```python
from build123d import *

# Parameters (mm, degrees)
BASE_FLANGE1_START                           = -50
BASE_FLANGE1_DEPTH                           = 100
CSK_FOR_M5_COUNTERSUNK_FLAT_HEAD_SCR_2_COUNT = 2
CSK_FOR_M5_COUNTERSUNK_FLAT_HEAD_SCR_2_PITCH = 50
FILLET1_R                                    = 10


# Read off the part's stored shape, not the designer's step: Base-Flange1
with BuildPart() as part:
    # Base-Flange1 outline → Base-Flange1 (new body)
    with BuildSketch(Plane(origin=(0, 0, 0), x_dir=(0, 0, -1), z_dir=(1, 0, 0)).offset(BASE_FLANGE1_START)):
        with BuildLine():
            Line((-47.884076231, -4), (50, -4))
            Line((50, -4), (50, 0))
            Line((50, 0), (-47.884076231, 0))
            ThreePointArc((-47.884076231, 0), (-49.967854363, -0.182306964), (-51.988317951, -0.723688551))
            Line((-51.988317951, -0.723688551), (-100, -18.198511713))
            Line((-100, -18.198511713), (-98.631919427, -21.957282196))
            Line((-98.631919427, -21.957282196), (-50.620237378, -4.482459034))
            ThreePointArc((-50.620237378, -4.482459034), (-49.273261653, -4.121537976), (-47.884076231, -4))
        make_face()
    extrude(amount=BASE_FLANGE1_DEPTH)

    # Sketch8 → CSK for M5 Countersunk Flat Head Screw1 (revolve, cut)
    with BuildSketch(Plane(origin=(0, -4, 25), x_dir=(0, 0, -1), z_dir=(1, 0, 0))):
        Polygon((0, 0), (0, 4), (2.75, 4), (2.75, 3.25), (6, 0), align=None)
    csk_for_m5_countersunk_flat_head_screw1 = revolve(axis=Axis((0, -10.35, 25), (0, 1, 0)), mode=Mode.SUBTRACT)

    # CSK for M5 Countersunk Flat Head Scr 2: CSK for M5 Countersunk Flat Head Screw1 ×2
    with Locations(*[(0, 0, -i * CSK_FOR_M5_COUNTERSUNK_FLAT_HEAD_SCR_2_PITCH) for i in range(1, CSK_FOR_M5_COUNTERSUNK_FLAT_HEAD_SCR_2_COUNT)]):
        add(csk_for_m5_countersunk_flat_head_screw1, mode=Mode.SUBTRACT)

    # Fillet1
    fillet1_edges = [part.edges().sort_by_distance(p)[0] for p in [
        (50, -20.077896954, 99.315959714),
        (50, -2, -50),
        (-50, -20.077896954, 99.315959714),
        (-50, -2, -50),
    ]]
    fillet(fillet1_edges, radius=FILLET1_R)


solid = part.part
```
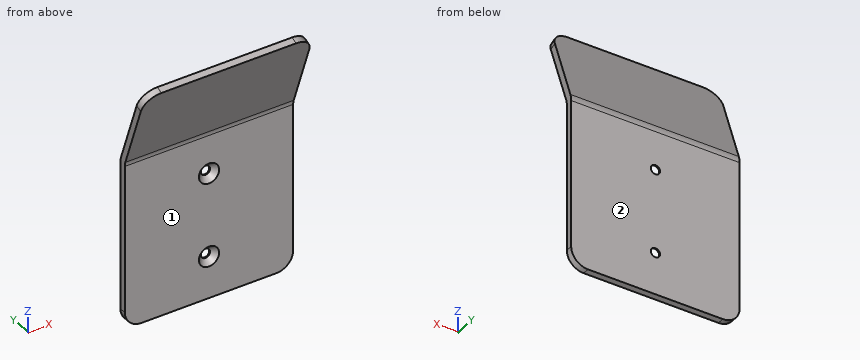
Input: part model. Units: mm. Frame: model coordinates. Face numbers are marked on the shaded views. A direction names the side the tool comes from. Give positions to 0.01 mm unless a question says otherwise; leave off trailing zeros. Loops run counter-clockwise (first coordinate to the right, second up) from the corner with the lowest first, then second, coordinate; pieces in that order, holes last.
1) Section query C-C on x = -31.5. Return the cut outline in (y, z), and give its area (3 significant figures).
A:
outline: (-21.96, 98.63) - (-4.48, 50.62) arc R8 cw to (-4, 47.88) - (-4, -50) - (0, -50) - (0, 47.88) arc R12 ccw to (-0.72, 51.99) - (-18.2, 100) - close
area: 610 mm2
2) Section query A-A on x = 0. Return the cut outline in (y, z).
A:
outline: (-21.96, 98.63) - (-4.48, 50.62) arc R8 cw to (-4, 47.88) - (-4, 31) - (-0.75, 27.75) - (0, 27.75) - (0, 47.88) arc R12 ccw to (-0.72, 51.99) - (-18.2, 100) - close; (-4, -50) - (0, -50) - (0, -27.75) - (-0.75, -27.75) - (-4, -31) - close; (-4, -19) - (-0.75, -22.25) - (0, -22.25) - (0, 22.25) - (-0.75, 22.25) - (-4, 19) - close
3) Contact query for flat-ended pins moving along their axis: pin 1 (12 mm diameter, centred on x = -39.5, z = -13.5, fed in from -Y); pin 2 (1.5 mm diameter, centred on x = -13.5, z = 71.5, fed in from -Y); pin 3 (6 mm diameter, centred on x = -22.5, z = 50.5, fed in from -Y); pin 4 (1 mm diameter, centred on y = -5, z = -33, fed in from +X). Output: stop coordinate, or through.
A:
pin 1: stops at y = -4
pin 2: stops at y = -12.36
pin 3: stops at y = -5.53
pin 4: passes through
4) Line query: L1, parallel to Y at x = 9, z = -23.5; L2, parallel to X at y = -0.35, z = -25; L3, parallel to X at y = -17, z = 92. Output: solid intervals per line, ascending.
A:
L1: y = -4 to 0
L2: x = -50 to -2.75, 2.75 to 50
L3: x = -49.78 to 49.78
5) Section query B-B on z = -25. Return the cut outline in (x, y), and give its area (3 significant figures).
A:
outline: (-50, -4) - (-6, -4) - (-2.75, -0.75) - (-2.75, 0) - (-50, 0) - close; (2.75, -0.75) - (6, -4) - (50, -4) - (50, 0) - (2.75, 0) - close
area: 367 mm2
6) Section query D-D on y = -9.75. Return the cut outline in (x, z), and give its area (3 significant figures).
A:
outline: (-50, 65.09) - (50, 65.09) - (50, 76.79) - (-50, 76.79) - close
area: 1,170 mm2
7) Reachability of the marked faces 1 and 2 from +Z, -Z, +X, -X, +Y, -Y: full face, straight path, thin tool, end or side. Return the list, or none.
A:
face 1: -Z, +X, -X, -Y
face 2: +Z, -Z, +X, -X, +Y
